Can you work these out from the drawing? Everything is in mm from the part's minimum corner. A direction names the side the tool comes from. Round coordinates to 2 decimals unless told otherwise and drop trailing zeros. Write each loop counter-clockwise with the first axis right and the second up, starting at its lowest first coordinate (ties: lowest second). Pieces come first, ordered by that corner, then holes. Notation, with made-up numbers: (-6, -8) - (52, -8) arc R24 ccw to (52, 8) - close; hole circle Ø11 at (73, -28.75). An arc over 180 degrees is marked (long way). One line per item, written item: value. Start each with the question number.
Item 1: Imagine slicing it at B-B, the plane x = 152.4. Please give me the cut outline in (y, z), then the cut area to 3 significant figures.
Item 2: Imagine slicing it at C-C, the plane z = 60. Count the separate pieces of the cut face and the enclosed holes in it, then the cut area to 3 significant figures.
Item 3: For P1, Ø14, axis at x = 153, y = 282, coming from the +Z side; P2, Ø12, axis at x = 261, z = 71.5, coming from the +Y side; P3, Ø6, axis at x = 267.5, y = 148, coming from the +Z side, each with a flat end and sliding along its axis, tell me the tip position at first contact or that it passes through.
Item 4: Imagine slicing it at D-D, the plane z = 106. Please give me the cut outline in (x, y), then the cut area to 3 significant figures.
Item 5: If I drill on line 1 (Z direction, x = 160, y = 79); line 2 (Y direction, x = 149, z = 36); line 3 (X direction, y = 172, z = 9), over which ranges is the centre line in solid material (lowest first)?
Item 6: For the marked faces 1 and 2, which set-ups out of +Z, -Z, +X, -X, +Y, -Y let a thin tool reach every point of the face, with its end or its side?
Item 7: Imagine slicing it at A-A, the plane y = 152.4. Please give me the cut outline in (x, z), then the cut area to 3 significant figures.
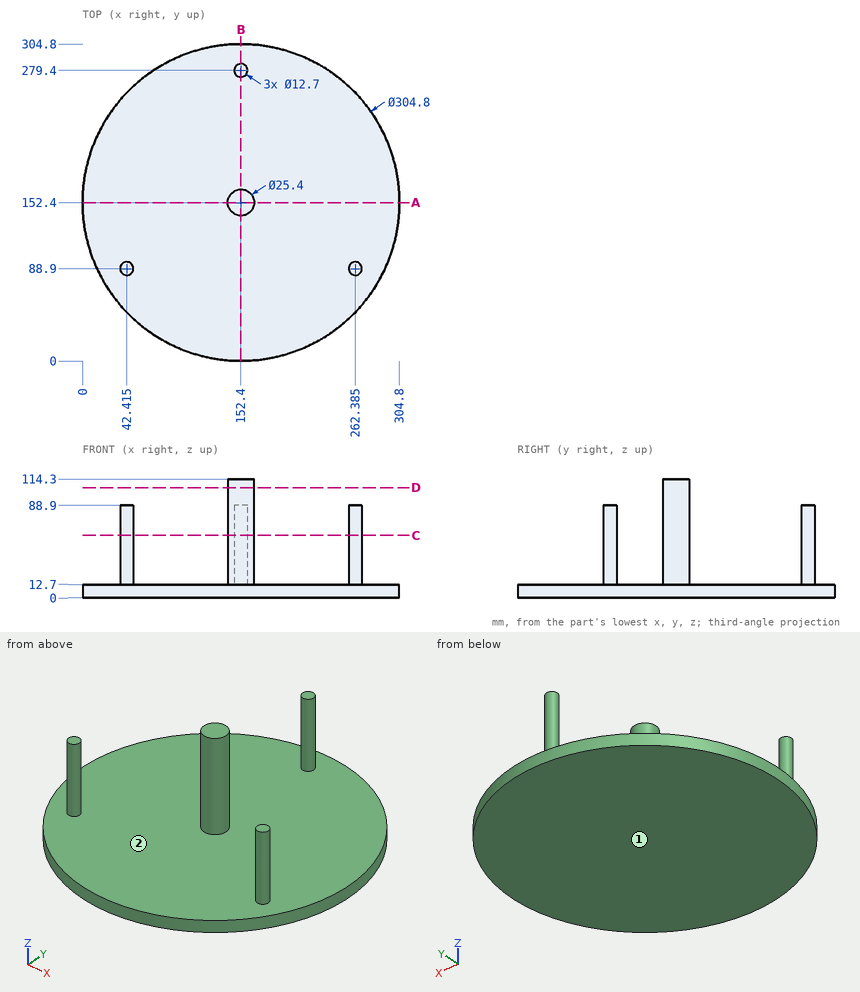
Values follow:
1. outline: (0, 0) - (304.8, 0) - (304.8, 12.7) - (285.75, 12.7) - (285.75, 88.9) - (273.05, 88.9) - (273.05, 12.7) - (165.1, 12.7) - (165.1, 114.3) - (139.7, 114.3) - (139.7, 12.7) - (0, 12.7) - close
1. area: 7,420 mm^2
2. separate pieces: 4
2. enclosed holes: 0
2. area: 887 mm^2
3. P1: stops at z = 88.9
3. P2: stops at y = 95.25
3. P3: stops at z = 12.7
4. outline: circle Ø25.4 at (152.4, 152.4)
4. area: 507 mm^2
5. line 1: z = 0 to 12.7
5. line 2: y = 140.16 to 164.64, 274.04 to 284.76
5. line 3: x = 1.27 to 303.53
6. face 1: -Z, +X, -X, +Y, -Y
6. face 2: +Z
7. outline: (0, 0) - (304.8, 0) - (304.8, 12.7) - (165.1, 12.7) - (165.1, 114.3) - (139.7, 114.3) - (139.7, 12.7) - (0, 12.7) - close
7. area: 6,450 mm^2
